Could you check a few things on this model? Use its own coordinates, in mm. Face numbers are marked on the shaded views. A direction names the side the tool comes from. Give positions to 0.01 mm unless a question says otherwise; leave off trailing zeros. Order: outer loops, then holes, each group sorted by start corner. A loop starts at its lowest first (then second) coordinate and runs counter-clockwise, first axis right, second up. Notation, with made-up numbers: (40, 16) -> (44, 16) arc R9 ccw to (44, 31) -> close; hole circle Ø2 at (49, 76.5). An arc over 180 degrees is marked (long way). One line per item, written item: value.
```python
from build123d import *

# Parameters (mm, degrees)
BOSS_EXTRUDE1_DEPTH    = 15
CUT_EXTRUDE1_OUTLINE_R = 3.25
CUT_EXTRUDE1_DEPTH     = 10
CUT_EXTRUDE2_DEPTH     = 1
CUT_EXTRUDE3_REACH     = 56.03
SKETCH5_W              = 8
SKETCH5_H              = 7.5
CUT_EXTRUDE4_DEPTH     = 2.5
FILLET1_R              = 5
FILLET2_R              = 4
FILLET4_R              = 5
FILLET5_R              = 1


# Read off the part's stored shape, not the designer's step: Cut-Extrude1
with BuildPart() as part:
    # Sketch1 → Boss-Extrude1 (new body)
    with BuildSketch(Plane.XY):
        Polygon((0, -8), (0, -30), (8, -30), (8, -57.5), (-10, -57.5), (-10, -61), (12, -61), (12, -8), align=None)
    extrude(amount=BOSS_EXTRUDE1_DEPTH)

    # Cut-Extrude1 outline → Cut-Extrude1 (cut)
    with BuildSketch(Plane.YZ):
        with Locations((-16.5, 7.5)):
            Circle(CUT_EXTRUDE1_OUTLINE_R)
    extrude(amount=CUT_EXTRUDE1_DEPTH, mode=Mode.SUBTRACT)

    # Sketch4 → Cut-Extrude2 (cut)
    with BuildSketch(Plane(origin=(0, -57.5, 0), x_dir=(1, 0, 0), z_dir=(0, 1, 0))):
        with BuildLine():
            Line((-2, -3), (-10, -3))
            Line((-10, -3), (-10, -12))
            Line((-10, -12), (-2, -12))
            ThreePointArc((-2, -12), (2.5, -7.5), (-2, -3))
        make_face()
    extrude(amount=-CUT_EXTRUDE2_DEPTH, mode=Mode.SUBTRACT)

    # Sketch5 → Cut-Extrude3 (cut, up to next)
    with BuildSketch(Plane(origin=(0, -58.5, 0), x_dir=(1, 0, 0), z_dir=(0, 1, 0)), mode=Mode.PRIVATE) as cut_extrude3_sk1:
        with BuildLine():
            ThreePointArc((-2, -11.25), (1.75, -7.5), (-2, -3.75))
            Line((-2, -3.75), (-2, -11.25))
        make_face()
    cut_extrude3_tool1 = extrude(cut_extrude3_sk1.sketch, amount=-CUT_EXTRUDE3_REACH, mode=Mode.PRIVATE) & part.part
    # Sketch5 → Cut-Extrude3 (cut, up to next)
    with BuildSketch(Plane(origin=(0, -58.5, 0), x_dir=(1, 0, 0), z_dir=(0, 1, 0)), mode=Mode.PRIVATE) as cut_extrude3_sk2:
        with Locations((-6, -7.5)):
            Rectangle(SKETCH5_W, SKETCH5_H)
    cut_extrude3_tool2 = extrude(cut_extrude3_sk2.sketch, amount=-CUT_EXTRUDE3_REACH, mode=Mode.PRIVATE) & part.part
    add(cut_extrude3_tool1.solids().sort_by_distance((-0.408451, -58.5, 7.5))[0], mode=Mode.SUBTRACT)
    add(cut_extrude3_tool2.solids().sort_by_distance((-6, -58.5, 7.5))[0], mode=Mode.SUBTRACT)

    # Sketch6 → Cut-Extrude4 (cut)
    with BuildSketch(Plane(origin=(0, -57.5, 0), x_dir=(1, 0, 0), z_dir=(0, 1, 0))):
        with BuildLine():
            Line((5.25, -7.5), (6.25, -7.5))
            ThreePointArc((6.25, -7.5), (6.215550668, -6.74685511), (6.11249037, -6))
            Line((6.11249037, -6), (5.25, -6))
            Line((5.25, -6), (5.25, -7.5))
        make_face()
        with BuildLine():
            ThreePointArc((6.11249037, -9), (6.215550668, -8.25314489), (6.25, -7.5))
            Line((6.25, -7.5), (5.25, -7.5))
            Line((5.25, -7.5), (5.25, -9))
            Line((5.25, -9), (6.11249037, -9))
        make_face()
    extrude(amount=-CUT_EXTRUDE4_DEPTH, mode=Mode.SUBTRACT)

    # Fillet1
    fillet1_edges = [part.edges().sort_by_distance(p)[0] for p in [
        (0, -30, 7.5),
    ]]
    fillet(fillet1_edges, radius=FILLET1_R)

    # Fillet2
    fillet2_edges = [part.edges().sort_by_distance(p)[0] for p in [
        (8, -30, 7.5),
    ]]
    fillet(fillet2_edges, radius=FILLET2_R)

    # Fillet4
    fillet4_edges = [part.edges().sort_by_distance(p)[0] for p in [
        (6, -8, 0),
        (6, -8, 15),
    ]]
    fillet(fillet4_edges, radius=FILLET4_R)

    # Fillet5
    fillet5_edges = [part.edges().sort_by_distance(p)[0] for p in [
        (8, -57.5, 7.5),
    ]]
    fillet(fillet5_edges, radius=FILLET5_R)


solid = part.part
```
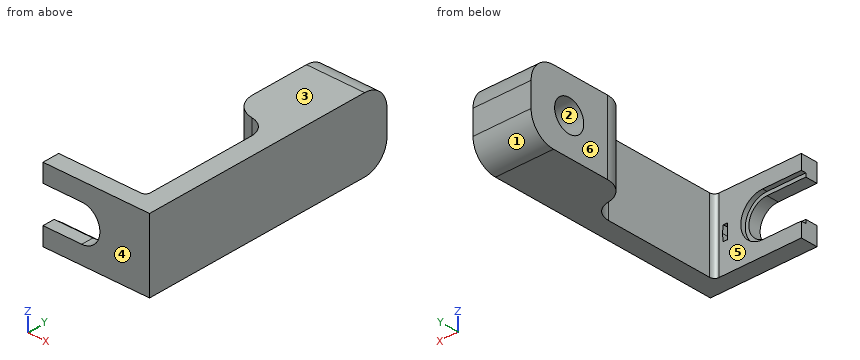
1) For P1, Ø4, axis at y = -30, z = 13.5, coming from the -X side; P2, Ø7, axis at y = -15.5, z = 8, coming from the -X side; P3, Ø4.5, axis at y = -44.5, z = 4, coming from the -X side; P4, Ø2.5, axis at x = -2, z = 9.5, coming from the +Y side, each with a flat end and sliding along its axis, tell me the tip position at first contact or that it passes through.
Answer below:
P1: stops at x = 1
P2: stops at x = 0
P3: stops at x = 8
P4: passes through
2) Suppose I cut it at A-A, the plane x = -2.75. Write out the boundary of the cut face in (y, z).
Answer below:
outline: (-61, 0) -> (-57.5, 0) -> (-57.5, 3) -> (-58.5, 3) -> (-58.5, 3.75) -> (-61, 3.75) -> close; (-61, 11.25) -> (-58.5, 11.25) -> (-58.5, 12) -> (-57.5, 12) -> (-57.5, 15) -> (-61, 15) -> close
3) Suppose I cut it at C-C, the plane y = -35. Write out the boundary of the cut face in (x, z).
Answer below:
outline: (8, 0) -> (12, 0) -> (12, 15) -> (8, 15) -> close
4) For the marked faces 4, 5 and 6, which set-ups out of +Z, -Z, +X, -X, +Y, -Y let a thin tool reach every point of the face, with its end or its side?
Answer below:
face 4: +Z, -Z, +X, -X, -Y
face 5: +Z, -Z, -X
face 6: +Z, -Z, -X, +Y
5) If I drill on line 1 along Y through (x, z) = (2.75, 9.5); line 2 along Z through (x, y) = (5.25, -16.5); line 3 along Y through (x, z) = (5, 7.25), over which ranges is the centre line in solid material (lowest first)?
Answer below:
line 1: y = -61 to -57.5, -29.47 to -19.06, -13.94 to -8
line 2: z = 0 to 4.25, 10.75 to 15
line 3: y = -61 to -57.5, -30.07 to -19.74, -13.26 to -8
6) We'd pull the mould along Y, two halves only. Please class the marked faces 1, 2 and 3: +Y half, -Y half, draft (parallel to the pull), parting line (faces both ways), or undercut.
Answer below:
face 1: +Y half
face 2: undercut
face 3: draft
7) Suppose I cut it at B-B, the plane y = -16.5. Write out the boundary of the cut face in (x, z), then the cut area to 3 significant figures.
Answer below:
outline: (0, 0) -> (12, 0) -> (12, 15) -> (0, 15) -> (0, 10.75) -> (10, 10.75) -> (10, 4.25) -> (0, 4.25) -> close
area: 115 mm2
